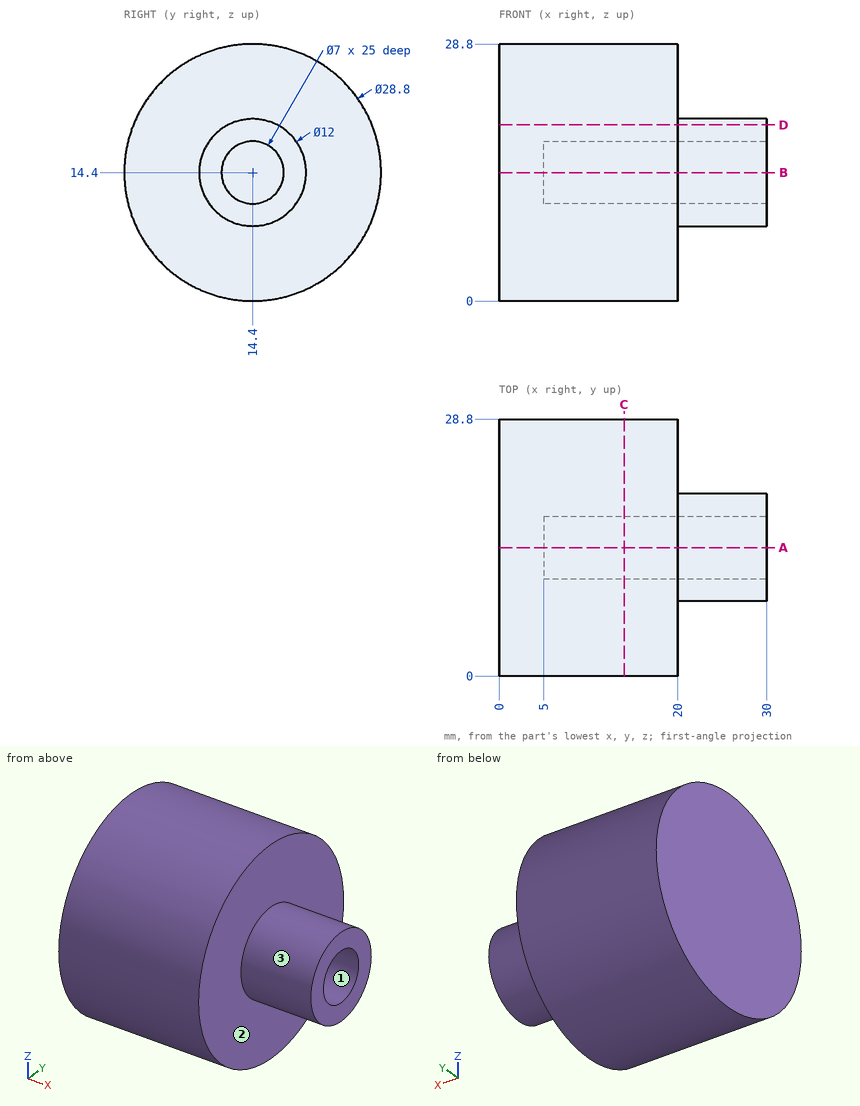
Drawing for the job (mm, zero at the part's lowest x, y, z). Give positions to 0.01 mm unless a question says otherwise; leave off trailing zeros. Loops run counter-clockwise (first coordinate to the right, second up) from the corner with the lowest first, then second, coordinate; pieces in that order, holes last. Notation, with made-up numbers: (-38, -36) - (5, -36) arc R16 ccw to (5, -24) - close; hole circle Ø5 at (74, 82). An arc over 180 degrees is marked (long way). Write item = value, one per line. Start each with the question number.
1) Band-saw the part on C-C on x = 14. Give the cut face in (y, z), plus the area to 3 significant figures.
2) Pull direction Z, two halves, no side cores. Call the marked faces 1, 2 and 3: +Z half, -Z half, draft (parallel to the pull), parting line (faces both ways), or undercut.
3) Drop flat-ended pins along their axis: pin 1 Ø2 at (y, z) = (23.5, 19.5) entering from -X; pin 2 Ø6 at (x, y) = (15.5, 18.5) entering from -Z; pin 3 Ø3 at (x, y) = (8.5, 19.5) entering from +Z; pin 4 Ø6 at (y, z) = (6, 20) entering from +X. Give the stop position or say it passes through.
4) Band-saw the part on D-D on z = 19.75. Give the cut face in (x, y).
5) Band-saw the part on A-A on y = 14.4. Give the cut face in (x, z).
6) Probe probe 1 along Y at (x, z) = (20.5, 14.4); probe 2 along X at (y, z) = (13.5, 14.75); probe 3 along X at (y, z) = (20.75, 23.5). List the from-to ranges inside material, lowest first. Write a range as from..to.
Final values:
q1.outline = circle Ø28.8 at (14.4, 14.4); hole circle Ø7 at (14.4, 14.4)
q1.area = 613 mm²
q2.face_1 = undercut
q2.face_2 = draft
q2.face_3 = parting line
q3.pin_1 = 0
q3.pin_2 = 0.04
q3.pin_3 = 28.34
q3.pin_4 = 20
q4.outline = (0, 1.03) - (20, 1.03) - (20, 11.68) - (30, 11.68) - (30, 17.12) - (20, 17.12) - (20, 27.77) - (0, 27.77) - close
q5.outline = (0, 0) - (20, 0) - (20, 8.4) - (30, 8.4) - (30, 10.9) - (5, 10.9) - (5, 17.9) - (30, 17.9) - (30, 20.4) - (20, 20.4) - (20, 28.8) - (0, 28.8) - close
q6.probe_1 = 8.4..10.9, 17.9..20.4
q6.probe_2 = 0..5
q6.probe_3 = 0..20
